Verification items for the finished model (mm, model axes). A direction names the side the tool comes from. Round coordinates to 2 decimals unless told otherwise and drop trailing zeros. Write each loop counter-clockwise with the first axis right and the second up, starting at its lowest first coordinate (ties: lowest second). Pieces come first, ordered by that corner, then holes. Notation, with made-up numbers: (39.5, 84.5) - (80.5, 84.5) arc R12 ccw to (80.5, 104.5) - close; hole circle Ø11 at (-15.5, 2). An arc over 180 degrees is marked (long way). Answer as a JSON object with one key per item and string values. Group by question number.
1) Section check C-C (x = 33.5). Enter the section's corners in (y, z) (1 decimal).
2) Section check A-A (y = 14). Enter the section's corners in (x, z) (1 decimal), then the cut area to 3 significant figures.
3) Set-up check for faces 1 (the flat face through (4, 41.275, 11)), 2 (the flat face through (23, 20, 4.762)): record each of +Z, -Z, +X, -X, +Y, -Y from which the full face is reachable in a straight line by a thin tool's end or side.
4) Go/stop test with flat-tipped pins: pin 1 Ø1 at (x, y) = (34, 36.5) entering from +Z; pin 2 Ø12.5 at (y, z) = (18, 20.5) entering from +X; pin 3 Ø10 at (x, y) = (11, 26) entering from +Z. Record where each tip stops, or that it passes through.
5) Thickness scan on line 1 (X direction, y = 28.5, z = 28); line 2 (Z direction, x = 36, y = 32.5). Record the ranges inside material, lowest first.
6) Section check B-B (z = 34.5). Enter the section's corners in (x, y) (1 decimal).
Solid Edge part; units mm, degrees
sketch "Sketch1" plane through (0, 0, 0) normal (0, -1, 0) x (1, 0, 0)
  line L0 (0, 38.1) -> (0, 0)
  line L1 (0, 0) -> (38.1, 0)
  line L2 (38.1, 0) -> (38.1, 1.905)
  arc A0 (38.1, 1.905) -> (35.2425, 4.7625) centre (35.2425, 1.905) ccw
  line L3 (35.2425, 4.7625) -> (10.4775, 4.7625)
  arc A1 (10.4775, 4.7625) -> (4.7625, 10.4775) centre (10.4775, 10.4775) cw
  line L4 (4.7625, 10.4775) -> (4.7625, 35.2425)
  arc A2 (4.7625, 35.2425) -> (1.905, 38.1) centre (1.905, 35.2425) ccw
  line L5 (1.905, 38.1) -> (0, 38.1)
extrude "Protrusion1" add sketch "Sketch1" against normal blind 41.275
Returned:
{
 "1": {"outline": "(0, 0) - (41.3, 0) - (41.3, 4.8) - (0, 4.8) - close"},
 "2": {"outline": "(0, 0) - (38.1, 0) - (38.1, 1.9) arc R2.9 ccw to (35.2, 4.8) - (10.5, 4.8) arc R5.7 cw to (4.8, 10.5) - (4.8, 35.2) arc R2.9 ccw to (1.9, 38.1) - (0, 38.1) - close", "area": "344 mm2"},
 "3": {"face 1": "+Z, -Z, +X, -X, +Y", "face 2": "+Z, +X, +Y, -Y"},
 "4": {"pin 1": "z = 4.76", "pin 2": "x = 4.76", "pin 3": "z = 6.93"},
 "5": {"line 1": "0 to 4.76", "line 2": "0 to 4.66"},
 "6": {"outline": "(0, 0) - (4.8, 0) - (4.8, 41.3) - (0, 41.3) - close"}
}
